Geometry check sheet. Reference: the model listing, model coordinates, mm. A direction names the side the tool comes from. Give positions to 0.01 mm unless a question says otherwise; leave off trailing zeros. Loops run counter-clockwise (first coordinate to the right, second up) from the corner with the lowest first, then second, coordinate; pieces in that order, holes last.
1. Tool access check on faces 1 (the flat face through (-73, 20, -63)), 2 (the flat face through (-24, 12, -66.722)). Record the directions out of +Z, -Z, +X, -X, +Y, -Y that give a thin tool (end or side, any length) a straight path to the whole face; none if there is none.
2. Go/stop test with flat-tipped pins: pin 1 Ø6 at (x, y) = (-80.5, 5) entering from -Z; pin 2 Ø4 at (x, y) = (-81, 15.5) entering from -Z; pin 3 Ø6.5 at (x, y) = (-67.82, 10.4) entering from -Z. Record where each tip stops, or that it passes through.
3. Cross-section at A-A, the plane y = 5. Record the cut outline in (x, z), plus the area to 4 significant figures.
4. Cross-section at B-B, the plane x = -53.5. Record the cut outline in (y, z).
5. Cross-section at C-C, the plane z = -92.5. Record the cut outline in (x, y).
6. Release check for a two-part mould opening along Y. For faces 3 (the cylindrical face through (-23.726, 10.49, -56.862)), 4 (the flat face through (-101, 10, -166.722)), 5 (the flat face through (-73, 0, -63)), 6 (the cylindrical face through (-69.827, 11.028, -56.862)) record: +Y half, -Y half, draft (parallel to the pull), parting line (faces both ways), or undercut.
7. Material ranges on L1, parallel to Z at x = 7, y = 19; L2, parallel to X at y = 15, z = -132; L3, parallel to X at y = 10.25, z = -83, recorded low to high.
from build123d import *

# Parameters (mm, degrees)
BOSS_EXTRUDE1_DEPTH = 20
SKETCH2_R           = 2.1
CUT_EXTRUDE3_DEPTH  = 20


with BuildPart() as part:
    # Sketch1 → Boss-Extrude1 (new body)
    with BuildSketch(Plane(origin=(0, 0, 0), x_dir=(1, 0, 0), z_dir=(0, 1, 0))):
        with BuildLine():
            Line((23.176256614, 46.721781305), (-90.573743386, 46.721781305))
            ThreePointArc((-90.573743386, 46.721781305), (-104.71587901, 52.579645681), (-110.573743386, 66.721781305))
            Line((-110.573743386, 66.721781305), (-110.573743386, 166.721781305))
            Line((-110.573743386, 166.721781305), (-90.573743386, 166.721781305))
            Line((-90.573743386, 166.721781305), (-90.573743386, 86.721781305))
            ThreePointArc((-90.573743386, 86.721781305), (-84.71587901, 72.579645681), (-70.573743386, 66.721781305))
            Line((-70.573743386, 66.721781305), (23.176256614, 66.721781305))
            Line((23.176256614, 66.721781305), (23.176256614, 46.721781305))
        make_face()
    extrude(amount=BOSS_EXTRUDE1_DEPTH)

    # Sketch2 → Cut-Extrude3 (cut)
    with BuildSketch(Plane(origin=(0, 0, -66.721781305), x_dir=(-1, 0, 0), z_dir=(0, 0, -1))):
        with Locations((25.823743386, 10.397679773)):
            Circle(SKETCH2_R)
        with Locations((67.823743386, 10.397679773)):
            Circle(SKETCH2_R)
    extrude(amount=-CUT_EXTRUDE3_DEPTH, mode=Mode.SUBTRACT)


solid = part.part
Result:
1. face 1: +Z, -Z, +X, -X, +Y
1. face 2: -Z, +X, +Y, -Y
2. pin 1: stops at z = -71.46
2. pin 2: stops at z = -71.05
2. pin 3: stops at z = -66.73
3. outline: (-110.57, -166.72) - (-90.57, -166.72) - (-90.57, -86.72) arc R20 cw to (-70.57, -66.72) - (23.18, -66.72) - (23.18, -46.72) - (-90.57, -46.72) arc R20 ccw to (-110.57, -66.72) - close
3. area: 4,675 mm2
4. outline: (0, -66.72) - (20, -66.72) - (20, -46.72) - (0, -46.72) - close
5. outline: (-110.57, 0) - (-90.57, 0) - (-90.57, 20) - (-110.57, 20) - close
6. face 3: undercut
6. face 4: draft
6. face 5: -Y half
6. face 6: undercut
7. L1: z = -66.72 to -46.72
7. L2: x = -110.57 to -90.57
7. L3: x = -110.57 to -90.22
